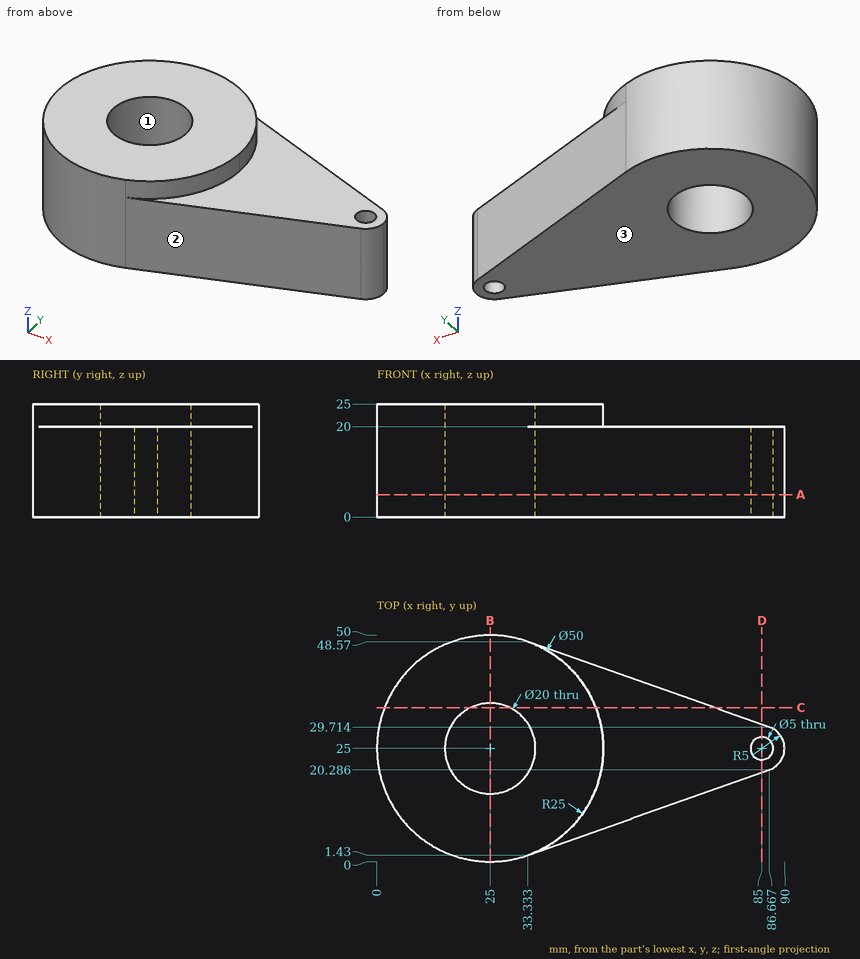
The figure shows three views and two pictorial views of one solid part (mm, origin at its lowest corner). Answer the questions. Give positions to 0.01 mm unless a question says otherwise; leave off trailing zeros. Order: outer loops, then holes, each group sorted by start corner. A loop starts at its lowest first (then second) coordinate and runs counter-clockwise, first axis right, second up. Notation, with made-up numbers: (3.25, 9.5) -> (38.25, 9.5) arc R34 ccw to (38.25, 40.5) -> close; hole circle Ø7 at (65.25, 24). An arc over 180 degrees is marked (long way). Answer as CSV lines item,"result". Start each with the question number.
(1) Consider line 1 along X through (y, z) = (25, 10); line 2 along Y through (x, z) = (25, 5.75); line 3 along Z through (x, y) = (63, 22.5). Determine where each line is inside the solid, lowest interval first.
(2) Section A-A, the plane z = 5 is taken. Write down the section's boundary in (x, y).
(3) Section B-B, the plane x = 25 is taken. Write down the section's boundary in (y, z), plus the area to 3 significant figures.
(4) Each of these flat-tipped pins is pushed along its axis until it touches: pin 1 Ø8 at (x, z) = (49, 14.5) entering from +Y (1 decimal); pin 2 Ø8 at (x, y) = (59.5, 30.5) entering from +Z; pin 3 Ø12 at (y, z) = (13, 3.5) entering from -X. Where does it stop, or does it pass through?
(5) Section C-C, the plane y = 34 is taken. Write down the section's boundary in (x, z).
(6) For a pull along Y with two mould halves and no side action, classify the marked faces 1, 2 and 3 as released by +Y, released by -Y, zero draft, split by the parting line, or undercut.
(7) Section D-D, the plane x = 85 is taken. Write down the section's boundary in (y, z), plus the area to 3 significant figures.
Entries:
1,line 1,"0 to 15, 35 to 82.5, 87.5 to 90"
1,line 2,"0 to 15, 35 to 50"
1,line 3,"0 to 20"
2,outline,"(33.33, 1.43) -> (86.67, 20.29) arc R5 ccw to (86.67, 29.71) -> (33.33, 48.57) arc R25 ccw (long way) to start; hole circle Ø20 at (25, 25); hole circle Ø5 at (85, 25)"
3,outline,"(0, 0) -> (15, 0) -> (15, 25) -> (0, 25) -> close; (35, 0) -> (50, 0) -> (50, 25) -> (35, 25) -> close"
3,area,"750 mm²"
4,pin 1,"y = 44.4"
4,pin 2,"z = 20"
4,pin 3,"x = 0.73"
5,outline,"(1.68, 0) -> (20.64, 0) -> (20.64, 25) -> (1.68, 25) -> close; (29.36, 0) -> (74.54, 0) -> (74.54, 20) -> (48.32, 20) -> (48.32, 25) -> (29.36, 25) -> close"
6,face 1,"undercut"
6,face 2,"released by -Y"
6,face 3,"zero draft"
7,outline,"(19.7, 0) -> (22.5, 0) -> (22.5, 20) -> (19.7, 20) -> close; (27.5, 0) -> (30.3, 0) -> (30.3, 20) -> (27.5, 20) -> close"
7,area,"112 mm²"
